Build history of the part. All positions in model axes, mm. Coordinates: 2 decimals unless noted, no trailing zeros. Loops run counter-clockwise (first coordinate to the right, second up) from the corner with the lowest first, then second, coordinate; pieces in that order, holes last.
(1) Slice it at D-D (z = 2.1). Give the number of separate pieces and of enclosed holes in the cut face, and give its area (3 significant figures).
(2) Wall check: L1, parallel to X at y = -14.5, z = 4; L2, parallel to Y at x = -21, z = 1.3; L3, parallel to X at y = -17, z = 1.7. Give the ranges that are in metal, low to high.
(3) Flat gauge pins, fed straight in: P1, Ø8, axis at x = -1, y = -9, coming from the -Z side; P2, Ø0.9, axis at x = -35.5, z = 1.5, coming from the -Y side. Where does each tip first touch, or does it go through?
(4) Slice it at B-B (x = -5.5). Give the cut face in (y, z).
(5) Slice it at A-A (y = 21.5). Give the cut face in (x, z), and give its area (3 significant figures).
(6) Slice it at C-C (y = 1). Give the cut face in (x, z), and give its area (3 significant figures).
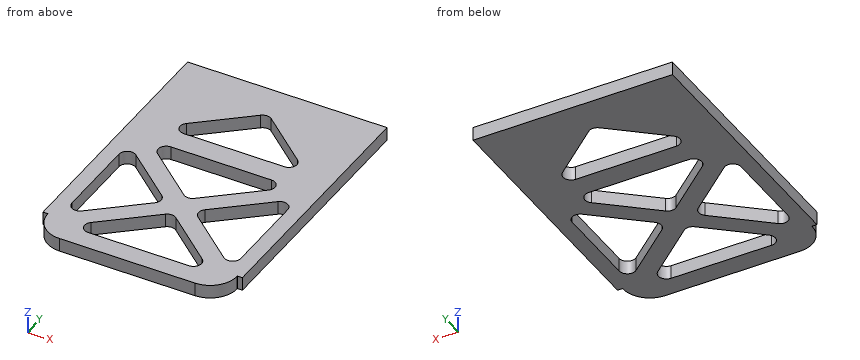
from build123d import *

# Parameters (mm, degrees)
SKETCH1_W           = 73.7
SKETCH1_H           = 105
BOSS_EXTRUDE1_DEPTH = 5
CUT_EXTRUDE1_REACH  = 68.392
CUT_EXTRUDE2_DEPTH  = 67.39218704


with BuildPart() as part:
    # Sketch1 → Boss-Extrude1 (new body)
    with BuildSketch(Plane.XY):
        with Locations((0, 2.5)):
            Rectangle(SKETCH1_W, SKETCH1_H)
    extrude(amount=BOSS_EXTRUDE1_DEPTH)

    # Sketch2 → Cut-Extrude1 (cut, up to next)
    with BuildSketch(Plane(origin=(0, 0, 0), x_dir=(-1, 0, 0), z_dir=(0, 0, -1)), mode=Mode.PRIVATE) as cut_extrude1_sk1:
        with BuildLine():
            Line((-18.606155591, -42.597211127), (18.606155591, -42.597211127))
            ThreePointArc((18.606155591, -42.597211127), (21.423509903, -40.627994657), (20.542210539, -37.30555425))
            Line((20.542210539, -37.30555425), (1.936054948, -21.586560733))
            ThreePointArc((1.936054948, -21.586560733), (0, -20.87821761), (-1.936054948, -21.586560733))
            Line((-1.936054948, -21.586560733), (-20.542210539, -37.30555425))
            ThreePointArc((-20.542210539, -37.30555425), (-21.423509903, -40.627994657), (-18.606155591, -42.597211127))
        make_face()
    cut_extrude1_tool1 = extrude(cut_extrude1_sk1.sketch, amount=-CUT_EXTRUDE1_REACH, mode=Mode.PRIVATE) & part.part
    # Sketch2 → Cut-Extrude1 (cut, up to next)
    with BuildSketch(Plane(origin=(0, 0, 0), x_dir=(-1, 0, 0), z_dir=(0, 0, -1)), mode=Mode.PRIVATE) as cut_extrude1_sk2:
        with BuildLine():
            Line((7.981018958, -17.791656877), (26.25814066, -33.232673486))
            ThreePointArc((26.25814066, -33.232673486), (29.457491922, -33.662060972), (31.194195607, -30.94101661))
            Line((31.194195607, -30.94101661), (31.194195607, -0.05898339))
            ThreePointArc((31.194195607, -0.05898339), (29.457491922, 2.662060972), (26.25814066, 2.232673486))
            Line((26.25814066, 2.232673486), (7.981018958, -13.208343123))
            ThreePointArc((7.981018958, -13.208343123), (6.917073906, -15.5), (7.981018958, -17.791656877))
        make_face()
    cut_extrude1_tool2 = extrude(cut_extrude1_sk2.sketch, amount=-CUT_EXTRUDE1_REACH, mode=Mode.PRIVATE) & part.part
    # Sketch2 → Cut-Extrude1 (cut, up to next)
    with BuildSketch(Plane(origin=(0, 0, 0), x_dir=(-1, 0, 0), z_dir=(0, 0, -1)), mode=Mode.PRIVATE) as cut_extrude1_sk3:
        with BuildLine():
            Line((-31.194195607, -0.05898339), (-31.194195607, -30.94101661))
            ThreePointArc((-31.194195607, -30.94101661), (-29.457491922, -33.662060972), (-26.25814066, -33.232673486))
            Line((-26.25814066, -33.232673486), (-7.981018958, -17.791656877))
            ThreePointArc((-7.981018958, -17.791656877), (-6.917073906, -15.5), (-7.981018958, -13.208343123))
            Line((-7.981018958, -13.208343123), (-26.25814066, 2.232673486))
            ThreePointArc((-26.25814066, 2.232673486), (-29.457491922, 2.662060972), (-31.194195607, -0.05898339))
        make_face()
    cut_extrude1_tool3 = extrude(cut_extrude1_sk3.sketch, amount=-CUT_EXTRUDE1_REACH, mode=Mode.PRIVATE) & part.part
    # Sketch2 → Cut-Extrude1 (cut, up to next)
    with BuildSketch(Plane(origin=(0, 0, 0), x_dir=(-1, 0, 0), z_dir=(0, 0, -1)), mode=Mode.PRIVATE) as cut_extrude1_sk4:
        with BuildLine():
            Line((18.606155591, 11.597211127), (-18.606155591, 11.597211127))
            ThreePointArc((-18.606155591, 11.597211127), (-21.423509903, 9.627994657), (-20.542210539, 6.30555425))
            Line((-20.542210539, 6.30555425), (-1.936054948, -9.413439267))
            ThreePointArc((-1.936054948, -9.413439267), (0, -10.12178239), (1.936054948, -9.413439267))
            Line((1.936054948, -9.413439267), (20.542210539, 6.30555425))
            ThreePointArc((20.542210539, 6.30555425), (21.423509903, 9.627994657), (18.606155591, 11.597211127))
        make_face()
    cut_extrude1_tool4 = extrude(cut_extrude1_sk4.sketch, amount=-CUT_EXTRUDE1_REACH, mode=Mode.PRIVATE) & part.part
    # Sketch2 → Cut-Extrude1 (cut, up to next)
    with BuildSketch(Plane(origin=(0, 0, 0), x_dir=(-1, 0, 0), z_dir=(0, 0, -1)), mode=Mode.PRIVATE) as cut_extrude1_sk5:
        with BuildLine():
            Line((18.606155591, 20), (-18.606155591, 20))
            ThreePointArc((-18.606155591, 20), (-21.423509903, 21.96921647), (-20.542210539, 25.291656877))
            Line((-20.542210539, 25.291656877), (-1.936054948, 41.010650393))
            ThreePointArc((-1.936054948, 41.010650393), (0, 41.718993517), (1.936054948, 41.010650393))
            Line((1.936054948, 41.010650393), (20.542210539, 25.291656877))
            ThreePointArc((20.542210539, 25.291656877), (21.423509903, 21.96921647), (18.606155591, 20))
        make_face()
    cut_extrude1_tool5 = extrude(cut_extrude1_sk5.sketch, amount=-CUT_EXTRUDE1_REACH, mode=Mode.PRIVATE) & part.part
    add(cut_extrude1_tool1.solids().sort_by_distance((0, -34.791369, 0))[0], mode=Mode.SUBTRACT)
    add(cut_extrude1_tool2.solids().sort_by_distance((-22.387881, -15.5, 0))[0], mode=Mode.SUBTRACT)
    add(cut_extrude1_tool3.solids().sort_by_distance((22.387881, -15.5, 0))[0], mode=Mode.SUBTRACT)
    add(cut_extrude1_tool4.solids().sort_by_distance((0, 3.791369, 0))[0], mode=Mode.SUBTRACT)
    add(cut_extrude1_tool5.solids().sort_by_distance((0, 27.805842, 0))[0], mode=Mode.SUBTRACT)

    # Sketch7 → Cut-Extrude2 (cut, through all)
    with BuildSketch(Plane.XY.offset(5)):
        with BuildLine():
            Line((-36.85, -39.9), (-36.85, -50))
            Line((-36.85, -50), (-25, -50))
            ThreePointArc((-25, -50), (-32.071067812, -47.071067812), (-35, -40))
            Line((-35, -40), (-35, -39.9))
            Line((-35, -39.9), (-36.85, -39.9))
        make_face()
        with BuildLine():
            ThreePointArc((35, -40), (32.071067812, -47.071067812), (25, -50))
            Line((25, -50), (36.85, -50))
            Line((36.85, -50), (36.85, -39.9))
            Line((36.85, -39.9), (35, -39.9))
            Line((35, -39.9), (35, -40))
        make_face()
    extrude(amount=-CUT_EXTRUDE2_DEPTH, mode=Mode.SUBTRACT)


solid = part.part
Response values:
1. separate pieces: 1
1. enclosed holes: 5
1. area: 4,830 mm2
2. L1: x = -36.85 to -31.19, -7.09 to 7.09, 31.19 to 36.85
2. L2: y = -50 to -41.41, -37.79 to -28.79, -2.21 to 6.79, 10.41 to 21.19, 24.81 to 55
2. L3: x = -36.85 to -31.19, -7.32 to 7.32, 31.19 to 36.85
3. P1: stops at z = 0
3. P2: stops at y = -39.9
4. outline: (-50, 0) - (-42.6, 0) - (-42.6, 5) - (-50, 5) - close; (-24.6, 0) - (-6.4, 0) - (-6.4, 5) - (-24.6, 5) - close; (11.6, 0) - (20, 0) - (20, 5) - (11.6, 5) - close; (38, 0) - (55, 0) - (55, 5) - (38, 5) - close
5. outline: (-36.85, 0) - (-21.2, 0) - (-21.2, 5) - (-36.85, 5) - close; (21.2, 0) - (36.85, 0) - (36.85, 5) - (21.2, 5) - close
5. area: 156 mm2
6. outline: (-36.85, 0) - (-31, 0) - (-31, 5) - (-36.85, 5) - close; (-24.8, 0) - (-14.26, 0) - (-14.26, 5) - (-24.8, 5) - close; (14.26, 0) - (24.8, 0) - (24.8, 5) - (14.26, 5) - close; (31, 0) - (36.85, 0) - (36.85, 5) - (31, 5) - close
6. area: 164 mm2
